The listing builds one solid part. Answer for the finished solid, in the listing's coordinates (mm). Face numbers are marked on the shaded views. A direction names the side the tool comes from. Coordinates: 2 decimals unless noted, no trailing zeros. Order: outer loops, then holes, each group sorted by start corner. A loop starts at its lowest first (then second) coordinate and runs counter-clockwise, first axis right, second up. Notation, with made-up numbers: (-15.5, -20.5) -> (-5.5, -20.5) arc R10 ccw to (-5.5, -3.5) -> close; hole circle Ø9 at (19, 15.25). An arc over 180 degrees is marked (long way). Answer in a Markdown table with one row per item.
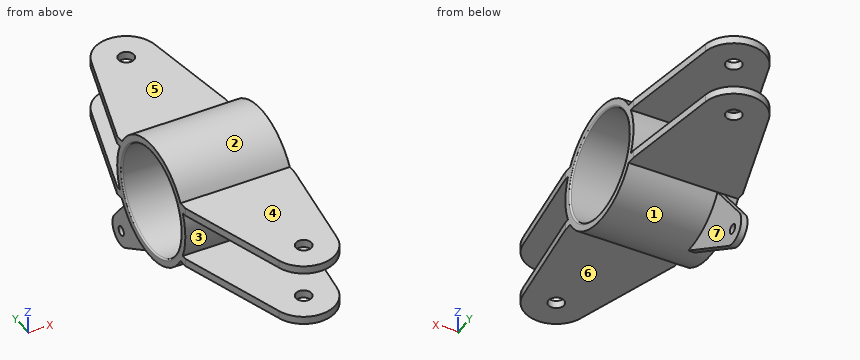
```python
from build123d import *

# Parameters (mm, degrees)
SKETCH1_R             = 39.007
SKETCH1_R_2           = 34.007
BOSS_EXTRUDE1_DEPTH   = 35
BOSS_EXTRUDE2_START   = 15
SKETCH2_R             = 5.007
BOSS_EXTRUDE2_DEPTH   = 5
BOSS_EXTRUDE2_2_DEPTH = 5
BOSS_EXTRUDE3_START   = -15
SKETCH3_R             = 5.007
BOSS_EXTRUDE3_DEPTH   = 5
BOSS_EXTRUDE3_2_DEPTH = 5
BOSS_EXTRUDE4_DEPTH   = 70
BOSS_EXTRUDE6_START   = -4
SKETCH6_R             = 3
BOSS_EXTRUDE6_DEPTH   = 4
FILLET1_R             = 1
FILLET2_R             = 1


with BuildPart() as part:
    # Sketch1 → Boss-Extrude1 (new, symmetric)
    with BuildSketch(Plane(origin=(0, 0, 0), x_dir=(0, 0, -1), z_dir=(1, 0, 0))):
        Circle(SKETCH1_R)
        Circle(SKETCH1_R_2, mode=Mode.SUBTRACT)
    extrude(amount=BOSS_EXTRUDE1_DEPTH, both=True)



with BuildPart() as body_2:
    # Sketch2 → Boss-Extrude2 (new body)
    with BuildSketch(Plane.XY.offset(BOSS_EXTRUDE2_START)):
        with BuildLine():
            Line((-35, -39.007), (35, -39.007))
            Line((35, -39.007), (25.596649495, -104.444761639))
            ThreePointArc((25.596649495, -104.444761639), (7.437713907, -121.532834549), (-13.266839867, -107.637848746))
            Line((-13.266839867, -107.637848746), (-35, -39.007))
        make_face()
        with Locations((5.8, -101.6)):
            Circle(SKETCH2_R, mode=Mode.SUBTRACT)
    extrude(amount=BOSS_EXTRUDE2_DEPTH)


with BuildPart() as body_3:
    # Sketch2 → Boss-Extrude2 2 (new body)
    with BuildSketch(Plane.XY.offset(BOSS_EXTRUDE2_START)):
        with BuildLine():
            Line((35, 39.007), (-35, 39.007))
            Line((-35, 39.007), (-13.266839867, 107.637848746))
            ThreePointArc((-13.266839867, 107.637848746), (7.437713907, 121.532834549), (25.596649495, 104.444761639))
            Line((25.596649495, 104.444761639), (35, 39.007))
        make_face()
        with Locations((5.8, 101.6)):
            Circle(SKETCH2_R, mode=Mode.SUBTRACT)
    extrude(amount=BOSS_EXTRUDE2_2_DEPTH)


with BuildPart() as body_4:
    # Sketch3 → Boss-Extrude3 (new body)
    with BuildSketch(Plane.XY.offset(BOSS_EXTRUDE3_START)):
        with BuildLine():
            Line((-35, -39.007), (-13.266839867, -107.637848746))
            ThreePointArc((-13.266839867, -107.637848746), (7.437713907, -121.532834549), (25.596649495, -104.444761639))
            Line((25.596649495, -104.444761639), (35, -39.007))
            Line((35, -39.007), (-35, -39.007))
        make_face()
        with Locations((5.8, -101.6)):
            Circle(SKETCH3_R, mode=Mode.SUBTRACT)
    extrude(amount=-BOSS_EXTRUDE3_DEPTH)


with BuildPart() as body_5:
    # Sketch3 → Boss-Extrude3 2 (new body)
    with BuildSketch(Plane.XY.offset(BOSS_EXTRUDE3_START)):
        with BuildLine():
            Line((-35, 39.007), (35, 39.007))
            Line((35, 39.007), (25.596649495, 104.444761639))
            ThreePointArc((25.596649495, 104.444761639), (7.437713907, 121.532834549), (-13.266839867, 107.637848746))
            Line((-13.266839867, 107.637848746), (-35, 39.007))
        make_face()
        with Locations((5.8, 101.6)):
            Circle(SKETCH3_R, mode=Mode.SUBTRACT)
    extrude(amount=-BOSS_EXTRUDE3_2_DEPTH)


with BuildPart() as part_1:
    add(part.part)

    add(body_2.part)  # Boss-Extrude4 merges body 2

    add(body_3.part)  # Boss-Extrude4 merges body 3

    add(body_4.part)  # Boss-Extrude4 merges body 4

    add(body_5.part)  # Boss-Extrude4 merges body 5
    # Sketch4 → Boss-Extrude4 (add)
    with BuildSketch(Plane(origin=(35, 0, 0), x_dir=(0, 0, -1), z_dir=(1, 0, 0))):
        with BuildLine():
            Line((20, -39.007), (15, -39.007))
            Line((15, -39.007), (15, -36.007583215))
            ThreePointArc((15, -36.007583215), (17.545232866, -34.838353186), (20, -33.489491621))
            Line((20, -33.489491621), (20, -39.007))
        make_face()
        with BuildLine():
            Line((-20, -39.007), (-15, -39.007))
            Line((-15, -39.007), (-15, -36.007583215))
            ThreePointArc((-15, -36.007583215), (-17.545232866, -34.838353186), (-20, -33.489491621))
            Line((-20, -33.489491621), (-20, -39.007))
        make_face()
        with BuildLine():
            Line((-20, 39.007), (-15, 39.007))
            Line((-15, 39.007), (-15, 36.007583215))
            ThreePointArc((-15, 36.007583215), (-17.545232866, 34.838353186), (-20, 33.489491621))
            Line((-20, 33.489491621), (-20, 39.007))
        make_face()
        with BuildLine():
            Line((20, 39.007), (15, 39.007))
            Line((15, 39.007), (15, 36.007583215))
            ThreePointArc((15, 36.007583215), (17.545232866, 34.838353186), (20, 33.489491621))
            Line((20, 33.489491621), (20, 39.007))
        make_face()
    extrude(amount=-BOSS_EXTRUDE4_DEPTH)

    # Sketch6 → Boss-Extrude6 (add)
    with BuildSketch(Plane.ZY.offset(25.9).offset(BOSS_EXTRUDE6_START)):
        with BuildLine():
            Line((-20, 33.489491621), (-50.098811723, 58.375353815))
            ThreePointArc((-50.098811723, 58.375353815), (-62.911300808, 58.318387785), (-65.151054806, 45.703054903))
            Line((-65.151054806, 45.703054903), (-39.007, 0))
            ThreePointArc((-39.007, 0), (-33.924077357, 19.253649641), (-20, 33.489491621))
        make_face()
        with Locations((-56.470917013, 50.668455984)):
            Circle(SKETCH6_R, mode=Mode.SUBTRACT)
    extrude(amount=BOSS_EXTRUDE6_DEPTH)

    # Fillet1
    fillet1_edges = [part_1.edges().sort_by_distance(p)[0] for p in [
        (35, 0, 34.007),
    ]]
    fillet(fillet1_edges, radius=FILLET1_R)

    # Fillet2
    fillet2_edges = [part_1.edges().sort_by_distance(p)[0] for p in [
        (-35, 0, 34.007),
    ]]
    fillet(fillet2_edges, radius=FILLET2_R)


solid = part_1.part
```
(1) For a pull along Z with two mould halves and no side action, classify the marked faces 1, 2 and 3 as released by +Z, released by -Z, zero draft, split by the parting line, or undercut.
Check values:
| item | result |
|---|---|
| face 1 | released by -Z |
| face 2 | released by +Z |
| face 3 | undercut |
(2) Flat-ended cylindrical pins translate along their axes: pin 1 (8 mm diameter, centred on x = -25, z = -27.5, fed in from +Y); pin 2 (14 mm diameter, centred on y = 42, z = -43.5, fed in from -X); pin 3 (1 mm diameter, centred on x = 27.5, z = -4.5, fed in from -Y). Find the tip coordinate at first contact, or state that the pin passes through.
Check values:
| item | result |
|---|---|
| pin 1 | y = 43 |
| pin 2 | x = -25.9 |
| pin 3 | y = -38.8 |
(3) A cutting plane is placed at D-D, the plane y = -60.5. Determine the outline of the cut face in (x, z), then the cut area to 3 significant figures.
Check values:
| item | result |
|---|---|
| outline | (-28.19, -20) -> (31.91, -20) -> (31.91, -15) -> (-28.19, -15) -> close; (-28.19, 15) -> (31.91, 15) -> (31.91, 20) -> (-28.19, 20) -> close |
| area | 601 mm² |
(4) A cutting plane is placed at C-C, the plane y = -101.6. Determine the outline of the cut face in (x, z).
Check values:
| item | result |
|---|---|
| outline | (-15.18, -20) -> (0.79, -20) -> (0.79, -15) -> (-15.18, -15) -> close; (-15.18, 15) -> (0.79, 15) -> (0.79, 20) -> (-15.18, 20) -> close; (10.81, -20) -> (26.01, -20) -> (26.01, -15) -> (10.81, -15) -> close; (10.81, 15) -> (26.01, 15) -> (26.01, 20) -> (10.81, 20) -> close |
(5) A cutting plane is placed at A-A, the plane x = 5.8. Count the separate pieces of the cut face and the enclosed holes in it, then the cut area to 3 significant figures.
Check values:
| item | result |
|---|---|
| separate pieces | 5 |
| enclosed holes | 1 |
| area | 2,680 mm² |
(6) Which of the six approach directions +Z, -Z, +X, -X, +Y, -Y give full straight-line access (tool end or side, diameter ignored) to the marked faces 4, 5, 6 and 7?
Check values:
| item | result |
|---|---|
| face 4 | +Z, +X, -X, -Y |
| face 5 | +Z, +X, -X, +Y |
| face 6 | -Z, +X, -X, -Y |
| face 7 | -Z, +X, +Y |
(7) Find the intervals of material crossed by line 1 along Z through (x, y) = (9.5, -70); line 2 along Y through (x, z) = (5, 18); line 3 along Y through (x, z) = (12, -1), in increasing order. Write a range as from..to.
Check values:
| item | result |
|---|---|
| line 1 | -20..-15, 15..20 |
| line 2 | -121.58..-106.54, -96.66..-28.85, 28.85..96.66, 106.54..121.58 |
| line 3 | -38.99..-33.99, 33.99..38.99 |
(8) A cutting plane is placed at B-B, the plane z = 0. Determine the outline of the cut face in (x, y).
Check values:
| item | result |
|---|---|
| outline | (-35, -39.01) -> (35, -39.01) -> (35, -35.01) arc R1 ccw to (34, -34.01) -> (-34, -34.01) arc R1 ccw to (-35, -35.01) -> close; (-35, 35.01) arc R1 ccw to (-34, 34.01) -> (34, 34.01) arc R1 ccw to (35, 35.01) -> (35, 39.01) -> (-35, 39.01) -> close |
